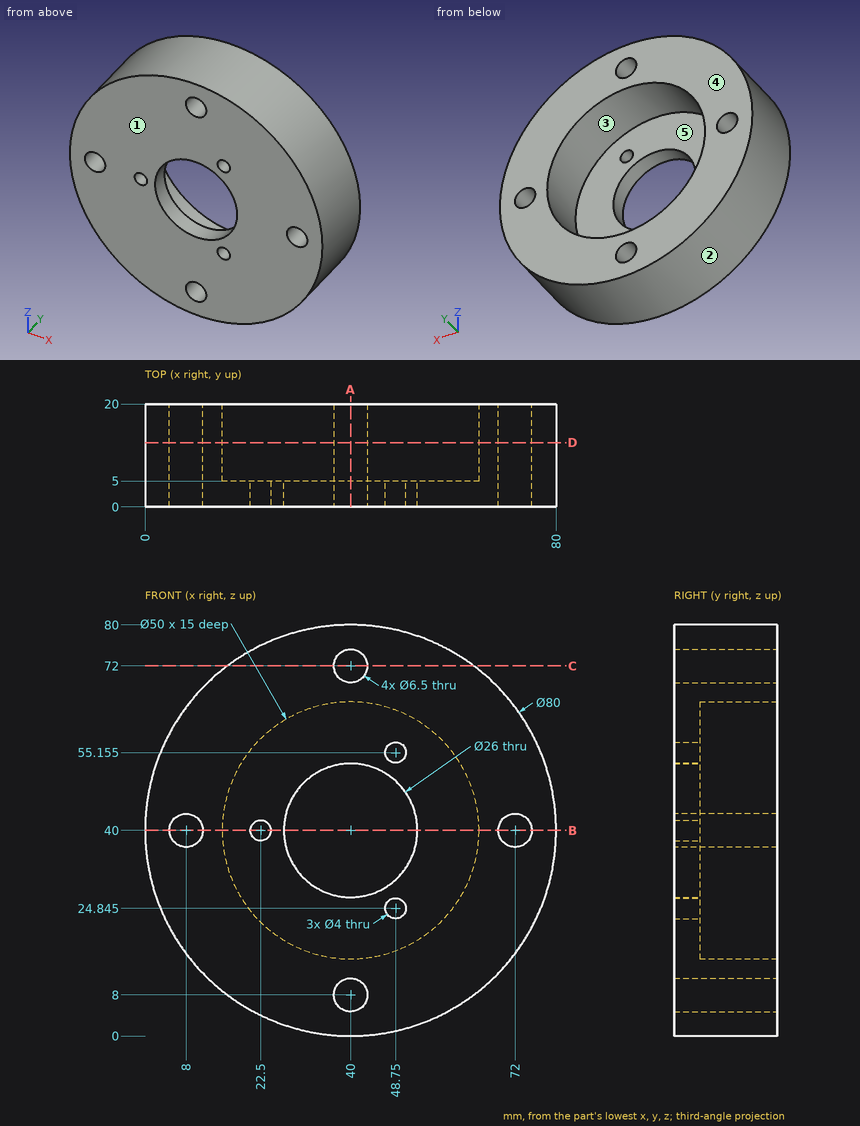
Design review of the part shown in the three views and the two pictorial views. Dimensions are in mm from the part's minimum x, y and z. A direction names the side the tool comes from. Coordinates: 2 decimals unless noted, no trailing zeros. Order: outer loops, then holes, each group sorted by start corner. A loop starts at its lowest first (then second) coordinate and runs counter-clockwise, first axis right, second up. Notation, with made-up numbers: (26, 47) - (68, 47) arc R6 cw to (68, 56) - close; hole circle Ø3 at (63.5, 82.25). An arc over 180 degrees is marked (long way). Answer as CSV lines item,"result". Start each with the question number.
1) Draft analysis for pull direction Z (two halves, no side actions). For the marked faces 1, 2 and 3, state which applies: +Z half, -Z half, draft (parallel to the pull), parting line (faces both ways), or undercut.
2) Machinability: for the marked faces 4 and 5, which of the approach directions +Z, -Z, +X, -X, +Y, -Y give a long, thin tool a straight path to every point of the face, cutting with its end or side? Answer none if there is none.
3) Add section C-C (z = 72). State the section outline as (x, y) points, then the cut area to 3 significant figures.
4) Add section A-A (x = 40). State the section outline as (y, z) points, then the cut area to 3 significant figures.
5) To check wall thickness, follow line 1 along Z through (x, y) = (40, 13.25); line 2 along Z through (x, y) = (48.75, 3.95) (1 decimal); line 3 along Y through (x, z) = (41, 24.5). State the ranges of each line that lie inside material, in increasing order. Write a range as [from, to].
6) Add section D-D (y = 12.5). State the section outline as (x, z) points, then the cut area to 3 significant figures.
7) Add section B-B (z = 40). State the section outline as (x, y) points, then the cut area to 3 significant figures.
8) Insertion check: P1, Ø1, axis at x = 43.5, z = 25, coming from the +Y side; P2, Ø8.5, axis at x = 40, z = 72, coming from the -Y side; P3, Ø8, axis at y = 17.5, z = 26.5, coming from the -X side (1 decimal); P4, Ø4, axis at y = 4, z = 37, coming from the +X side. Each pin has a flat end and moves straight along its axis. Give the tip position at first contact, or say it passes through.
Result:
1,face 1,"draft"
1,face 2,"parting line"
1,face 3,"undercut"
2,face 4,"+Z, -Z, +X, -X, +Y"
2,face 5,"+Y"
3,outline,"(16, 0) - (36.75, 0) - (36.75, 20) - (16, 20) - close; (43.25, 0) - (64, 0) - (64, 20) - (43.25, 20) - close"
3,area,"830 mm^2"
4,outline,"(0, 0) - (20, 0) - (20, 4.75) - (0, 4.75) - close; (0, 11.25) - (20, 11.25) - (20, 15) - (5, 15) - (5, 27) - (0, 27) - close; (0, 53) - (5, 53) - (5, 65) - (20, 65) - (20, 68.75) - (0, 68.75) - close; (0, 75.25) - (20, 75.25) - (20, 80) - (0, 80) - close"
4,area,"460 mm^2"
5,line 1,"[0, 4.75], [11.25, 15], [65, 68.75], [75.25, 80]"
5,line 2,"[1, 22.8], [26.8, 30.4], [49.6, 53.2], [57.2, 79]"
5,line 3,"[0, 5]"
6,outline,"circle Ø80 at (40, 40); hole circle Ø6.5 at (8, 40); hole circle Ø50 at (40, 40); hole circle Ø6.5 at (40, 8); hole circle Ø6.5 at (40, 72); hole circle Ø6.5 at (72, 40)"
6,area,"2,930 mm^2"
7,outline,"(0, 0) - (4.75, 0) - (4.75, 20) - (0, 20) - close; (11.25, 0) - (20.5, 0) - (20.5, 5) - (15, 5) - (15, 20) - (11.25, 20) - close; (24.5, 0) - (27, 0) - (27, 5) - (24.5, 5) - close; (53, 0) - (68.75, 0) - (68.75, 20) - (65, 20) - (65, 5) - (53, 5) - close; (75.25, 0) - (80, 0) - (80, 20) - (75.25, 20) - close"
7,area,"440 mm^2"
8,P1,"y = 5"
8,P2,"y = 0"
8,P3,"x = 1.1"
8,P4,"x = 79.99"
